Geometry: final body of the model. Coordinates: model frame, mm. A direction names the side the tool comes from. Coordinates: 2 decimals unless noted, no trailing zeros. Write each loop counter-clockwise with the first axis right and the second up, starting at its lowest first coordinate (ties: lowest second). Pieces come first, ordered by that corner, then holes.
from build123d import *

# Parameters (mm, degrees)
F1_DEPTH = 300
F2_W     = 100
F2_H     = 100
F3_DEPTH = 5
F5_D     = 8.8
F6_R     = 5
F7_R     = 5.1189485143
F8_DEPTH = 100


with BuildPart() as f1:
    # F0 (on Top) → F1 (new body, symmetric)
    with BuildSketch(Plane.XY):
        with BuildLine():
            Line((-31.5497371938, -15.77975575), (-25.5497371938, -15.77975575))
            Line((-25.5497371938, -15.77975575), (-25.5497371938, 18.2202439159))
            ThreePointArc((-25.5497371938, 18.2202439159), (-24.6710575374, 20.3415642595), (-22.5497371938, 21.2202439159))
            Line((-22.5497371938, 21.2202439159), (21.4502628062, 21.2202439159))
            ThreePointArc((21.4502628062, 21.2202439159), (23.5715831497, 20.3415642595), (24.4502628062, 18.2202439159))
            Line((24.4502628062, 18.2202439159), (24.4502628062, -15.77975575))
            Line((24.4502628062, -15.77975575), (30.4502628062, -15.77975575))
            Line((30.4502628062, -15.77975575), (30.4502628062, 24.2202439159))
            ThreePointArc((30.4502628062, 24.2202439159), (29.5715831497, 26.3415642595), (27.4502628062, 27.2202439159))
            Line((27.4502628062, 27.2202439159), (-28.5497371938, 27.2202439159))
            ThreePointArc((-28.5497371938, 27.2202439159), (-30.6710575374, 26.3415642595), (-31.5497371938, 24.2202439159))
            Line((-31.5497371938, 24.2202439159), (-31.5497371938, -15.77975575))
        make_face()
    extrude(amount=F1_DEPTH, both=True)

    # F2 (on Top) → F3 (join)
    with BuildSketch(Plane.XY):
        Rectangle(F2_W, F2_H)
    extrude(amount=F3_DEPTH)

    # F5 (through all)
    with Locations(Plane(origin=(-31.5497371938, 0, 0), x_dir=(0, -1, 0), z_dir=(-1, 0, 0))):
        with Locations((0.77975575, 280), (0.77975575, 65)):
            Hole(F5_D / 2)

    # F6
    f6_edges = [f1.edges().sort_by_distance(p)[0] for p in [
        (-28.549737, -15.779756, 300),
        (27.450263, -15.779756, 300),
    ]]
    fillet(f6_edges, radius=F6_R)

    # F7 (on Right) → F8 (join, symmetric)
    with BuildSketch(Plane.YZ):
        with Locations((6.0703633353, -269.5238888264)):
            Circle(F7_R)
    extrude(amount=F8_DEPTH, both=True)


solid = f1.part
Item 1: Section B-B, the plane z = -228.5. Output: boundary loops of the cut face in (x, y), plus the area to 3 significant figures.
Derived:
outline: (-31.55, -15.78) - (-25.55, -15.78) - (-25.55, 18.22) arc R3 cw to (-22.55, 21.22) - (21.45, 21.22) arc R3 cw to (24.45, 18.22) - (24.45, -15.78) - (30.45, -15.78) - (30.45, 24.22) arc R3 ccw to (27.45, 27.22) - (-28.55, 27.22) arc R3 ccw to (-31.55, 24.22) - close
area: 816 mm2
Item 2: Set-up query: faces 4 (the cylindrical face through (65.71, 5.4, -264.45)), 5 (the flat face through (-1, 1, 5)), 6 (the cylindrical face through (-65.3, 5.4, -264.45)). Return all of +Z, -Z, +X, -X, +Y, -Y with unobstructed straight access to the full face (end or side cutting, diameter ignored); none if empty.
Derived:
face 4: +X
face 5: +Z
face 6: -X
Item 3: Pull-direction query (Z, two-part tool) for faces 1 (the flat face through (-1, 21.22, -148)), 2 (the flat face through (-31.55, 5, -148)), 3 (the flat face through (-1, 22, 300)); classes: released by +Z, released by -Z, zero draft, split by the parting line, or undercut.
Derived:
face 1: zero draft
face 2: undercut
face 3: released by +Z
Item 4: Material intervals for probe 1 along X at (y, z) = (12, -271); probe 2 along Y at (x, z) = (27.6, 280); probe 3 along X at (y, z) = (22, -156), sorted ascending.
Derived:
probe 1: x = -31.55 to -25.55, 24.45 to 30.45
probe 2: y = -15.78 to -5.18, 3.62 to 27.22
probe 3: x = -31.55 to 30.45
Item 5: Section A-A, the plane x = 1.5. Output: boundary loops of the cut face in (y, z), plus the area to 3 significant figures.
Derived:
outline: (-50, 0) - (21.22, 0) - (21.22, -300) - (27.22, -300) - (27.22, 0) - (50, 0) - (50, 5) - (27.22, 5) - (27.22, 300) - (21.22, 300) - (21.22, 5) - (-50, 5) - close; circle Ø10.24 at (6.07, -269.52)
area: 4,150 mm2
Item 6: Section C-C, the plane y = -21. Output: boundary loops of the cut face in (x, z).
Derived:
outline: (-50, 0) - (50, 0) - (50, 5) - (-50, 5) - close
Item 7: Pin query (flat end, axial travel): pin 1 (5 mm diameter, centred on x = 27, z = 98, fed in from -Y); pin 2 (1.5 mm diameter, centred on x = -16.5, z = 153, fed in from -Y); pin 3 (10 mm diameter, centred on y = 1, z = -119.5, fed in from -X). Return the tip coordinate at first contact, or that it passes through.
Derived:
pin 1: stops at y = -15.78
pin 2: stops at y = 21.22
pin 3: stops at x = -31.55
